Build history of the part. All positions in model axes, mm. A direction names the side the tool comes from. Round coordinates to 2 decimals unless told otherwise and drop trailing zeros. Write each loop counter-clockwise with the first axis right and the second up, starting at its lowest first coordinate (ties: lowest second). Pieces come first, ordered by that corner, then holes. Notation, with made-up numbers: M -39,16.5 L -33,16.5 A12 cw -33,36.5 Z; hole C -35.75,16.5 d8. An arc over 180 degrees is marked long. Use a Markdown table: item, result.
from build123d import *

# Parameters (mm, degrees)
F1_W      = 200
F1_H      = 200
F2_DEPTH  = 100
F4_D      = 18.5
F4_DEPTH  = 22.5
F4_TIP    = 5.557960726
F5_SIZE   = 5
F6_R      = 5
F8_R      = 4.99999
F10_D     = 56
F10_DEPTH = 72
F10_TIP   = 16.8240973328


# Not quite as in the source:
# - a fillet or chamfer is up to 0.001 mm smaller than in the source, because OpenCascade refuses the exact size
# - a feature of the source that left no trace in its solid (it failed there, or was rolled back) is left out


with BuildPart() as f2:
    # F1 (on Front) → F2 (new body, symmetric)
    with BuildSketch(Plane.XZ):
        Rectangle(F1_W, F1_H)
    extrude(amount=F2_DEPTH, both=True)

    # F4
    with Locations(Plane.XZ.offset(100)):
        with Locations((0, 0)):
            Hole(F4_D / 2, depth=F4_DEPTH)
            with Locations((0, 0, -(F4_DEPTH + F4_TIP / 2))):  # 118° drill point
                Cone(0, F4_D / 2, F4_TIP, mode=Mode.SUBTRACT)

    # F5
    f5_edges = [f2.edges().sort_by_distance(p)[0] for p in [
        (0, -100, 100),
    ]]
    chamfer(f5_edges, length=F5_SIZE)

    # F6
    f6_edges = [f2.edges().sort_by_distance(p)[0] for p in [
        (100, 2.5, 100),
    ]]
    fillet(f6_edges, radius=F6_R)

    # F8 (radius 5 in the source; OpenCascade refuses exactly that, so slightly less here)
    f8_edges = [f2.edges().sort_by_distance(p)[0] for p in [
        (0, 100, -100),
        (-2.5, 100, 100),
        (98.535534, 100, 98.535534),
        (100, 100, -2.5),
        (100, -100, -2.5),
        (100, 0, -100),
    ]]
    fillet(f8_edges, radius=F8_R)

    # F10
    with Locations(Plane.XY.offset(100)):
        with Locations((0, 14.7048085928)):
            Hole(F10_D / 2, depth=F10_DEPTH)
            with Locations((0, 0, -(F10_DEPTH + F10_TIP / 2))):  # 118° drill point
                Cone(0, F10_D / 2, F10_TIP, mode=Mode.SUBTRACT)


solid = f2.part
Q1. Cut at A-A on z = 57. Give the cut face in (x, y), and give its area (3 significant figures).
Response values:
| item | result |
|---|---|
| outline | M -100,-100 L 95,-100 A5 ccw 100,-95 L 100,95 A5 ccw 95,100 L -100,100 Z; hole C 0,14.7 d56 |
| area | 37,500 mm2 |
Q2. Two-plate mould, pull along X, no slides. Class faces 3 (the cylindrical face through (2.01, -88.59, -9.03)), 4 (the flat face through (-4, 100, 1)), 5 (the flat face through (-100, -1, -1)): +X half, -X half, draft (parallel to the pull), parting line (faces both ways), or undercut.
Response values:
| item | result |
|---|---|
| face 3 | undercut |
| face 4 | draft |
| face 5 | -X half |
Q3. Which spindle directions (+Z, -Z, +X, -X, +Y, -Y) get a long thin tool onto all of the face, cutting with end or side? Do faces 1 (the cylindrical face through (3.645, 42.467, 63.496)), 2 (the flat face through (100, -1, -1)). Say none if no direction does.
Response values:
| item | result |
|---|---|
| face 1 | +Z |
| face 2 | +Z, -Z, +X, +Y, -Y |
Q4. Drop a flat-ended pin along its axis: P1, Ø16.5, axis at x = 0, z = 0, coming from the -Y side. Give the stop position or say it passes through.
Response values:
| item | result |
|---|---|
| P1 | stops at y = -76.9 |
Q5. Drill centre lines: L1, parallel to X at y = 13.5, z = 44.5; L2, parallel to X at y = -92, z = 0. Where is each one in solid material? Low to high.
Response values:
| item | result |
|---|---|
| L1 | x = -100 to -27.97, 27.97 to 100 |
| L2 | x = -100 to -9.25, 9.25 to 100 |
